```python
from build123d import *

# Parameters (mm, degrees)
BOSS_EXTRUDE1_DEPTH = 2.4


with BuildPart() as part:
    # Sketch2 → Boss-Extrude1 (new body)
    with BuildSketch(Plane(origin=(0, 0, 0), x_dir=(1, 0, 0), z_dir=(0, 1, 0))):
        with BuildLine():
            Line((25.28293267, 77.245611288), (22.241395548, 50.202851698))
            Line((22.241395548, 50.202851698), (15.224426897, 48.764665996))
            Line((15.224426897, 48.764665996), (21.775683691, 46.062138205))
            Line((21.775683691, 46.062138205), (20.878911595, 38.088803933))
            Line((20.878911595, 38.088803933), (25.3187138, 45.004925816))
            Line((25.3187138, 45.004925816), (29.758516004, 38.088803933))
            Line((29.758516004, 38.088803933), (28.861743908, 46.062138205))
            Line((28.861743908, 46.062138205), (35.413000702, 48.764665996))
            Line((35.413000702, 48.764665996), (28.396032051, 50.202851698))
            Line((28.396032051, 50.202851698), (25.354494929, 77.245611288))
            ThreePointArc((25.354494929, 77.245611288), (39.364716338, 50.558630658), (47.260701361, 21.470236759))
            ThreePointArc((47.260701361, 21.470236759), (43.131494569, 27.98329808), (38.487800716, 34.14011738))
            ThreePointArc((38.487800716, 34.14011738), (35.669967354, 35.788554713), (32.458155801, 35.203920598))
            ThreePointArc((32.458155801, 35.203920598), (15.517725775, 22.41503931), (1.838377838, 6.185156559))
            ThreePointArc((1.838377838, 6.185156559), (8.663390647, 43.331109422), (25.28293267, 77.245611288))
        make_face()
        with BuildLine():
            Line((28.761044533, 50.536354524), (25.936821585, 75.646941422))
            ThreePointArc((25.936821585, 75.646941422), (38.906137272, 50.63149335), (46.519959977, 23.502072134))
            ThreePointArc((46.519959977, 23.502072134), (42.849248676, 29.083132434), (38.797114504, 34.393741079))
            ThreePointArc((38.797114504, 34.393741079), (35.739465536, 36.182470951), (32.254308319, 35.548080741))
            ThreePointArc((32.254308319, 35.548080741), (15.763956049, 23.195791569), (2.309144184, 7.59198423))
            ThreePointArc((2.309144184, 7.59198423), (9.008069243, 43.099003198), (24.700606015, 75.646941422))
            Line((24.700606015, 75.646941422), (21.876383066, 50.536354524))
            Line((21.876383066, 50.536354524), (13.862415181, 48.893825592))
            Line((13.862415181, 48.893825592), (21.344500988, 45.807311742))
            Line((21.344500988, 45.807311742), (20.289917479, 36.430852681))
            Line((20.289917479, 36.430852681), (25.3187138, 44.264482803))
            Line((25.3187138, 44.264482803), (30.34751012, 36.430852681))
            Line((30.34751012, 36.430852681), (29.292926611, 45.807311742))
            Line((29.292926611, 45.807311742), (36.775012418, 48.893825592))
            Line((36.775012418, 48.893825592), (28.761044533, 50.536354524))
        make_face(mode=Mode.SUBTRACT)
    extrude(amount=BOSS_EXTRUDE1_DEPTH)


solid = part.part
```
For this review, take the finished solid that the model builds, in its own axes (mm). A direction names the side the tool comes from. Round coordinates to 2 decimals unless told otherwise and drop trailing zeros. Order: outer loops, then holes, each group sorted by start corner. A loop starts at its lowest first (then second) coordinate and runs counter-clockwise, first axis right, second up.
Q1. Machinability: for faces 5 (the flat face through (26.9, 1.2, -63.5)), 6 (the flat face through (31.4, 2.4, -49.8)), which of the approach directions +Z, -Z, +X, -X, +Y, -Y give a long, thin tool a straight path to every point of the face, cutting with its end or side? Answer none if there is none.
Findings below:
face 5: +Y, -Y
face 6: +Z, -Z, +X, -X, +Y
Q2. We need section D-D, the plane x = 44. Give the boundary of the cut face in (y, z).
Findings below:
outline: (0, -36.62) - (2.4, -36.62) - (2.4, -35.08) - (0, -35.08) - close; (0, -27.42) - (2.4, -27.42) - (2.4, -26.71) - (0, -26.71) - close
Q3. We need section A-A, the plane x = 23. Give the boundary of the cut face in (y, z), plus the area to 3 significant figures.
Findings below:
outline: (0, -73.74) - (2.4, -73.74) - (2.4, -72.99) - (0, -72.99) - close; (0, -60.53) - (2.4, -60.53) - (2.4, -56.95) - (0, -56.95) - close; (0, -41.39) - (2.4, -41.39) - (2.4, -40.65) - (0, -40.65) - close; (0, -29.31) - (2.4, -29.31) - (2.4, -28.8) - (0, -28.8) - close
area: 13.4 mm2
Q4. Insertion check: P1, Ø3, axis at x = 25, z = -49, coming from the -Y side; P2, Ø1, axis at x = 32.5, y = 0.5, coming from the +Z side; P3, Ø12, axis at x = 29.5, z = -48.5, coming from the +Y side. Each pin has a flat end and moves straight along its axis. Give the tip position at first contact, or say it passes through.
Findings below:
P1: passes through
P2: stops at z = -34.93
P3: stops at y = 2.4
Q5. Mouldability with a two-part tool opening along Z and no side actions: class faces 1 (the cylindrical face through (35.72, 1.18, -35.78)), 2 (the flat face through (23.07, 1.18, -41.5)), 3 (the cylindrical face through (8.5, 1.18, -42.83)), 4 (the flat face through (29.316, 1.183, -42.02)) as pulls with the +Z half, pulls with the -Z half, needs draft (parallel to the pull), parting line crosses it, or undercut.
Findings below:
face 1: pulls with the +Z half
face 2: undercut
face 3: pulls with the -Z half
face 4: undercut
Q6. Wall thickness on line 1 (X direction, y = 1.7, z = -60.5); line 2 (X direction, y = 0.65, z = -28); line 3 (Z direction, x = 35, y = 1.3): over which ranges is each line inside the solid? List them lowest first.
Findings below:
line 1: x = 15.64 to 16.08, 23 to 23.4, 27.24 to 27.64, 34.56 to 35
line 2: x = 4.56 to 4.97, 21.32 to 21.97, 43.12 to 43.61, 45.66 to 46.07
line 3: z = -60.5 to -59.58, -49.26 to -48.85, -48.59 to -48.16, -36.26 to -35.86
